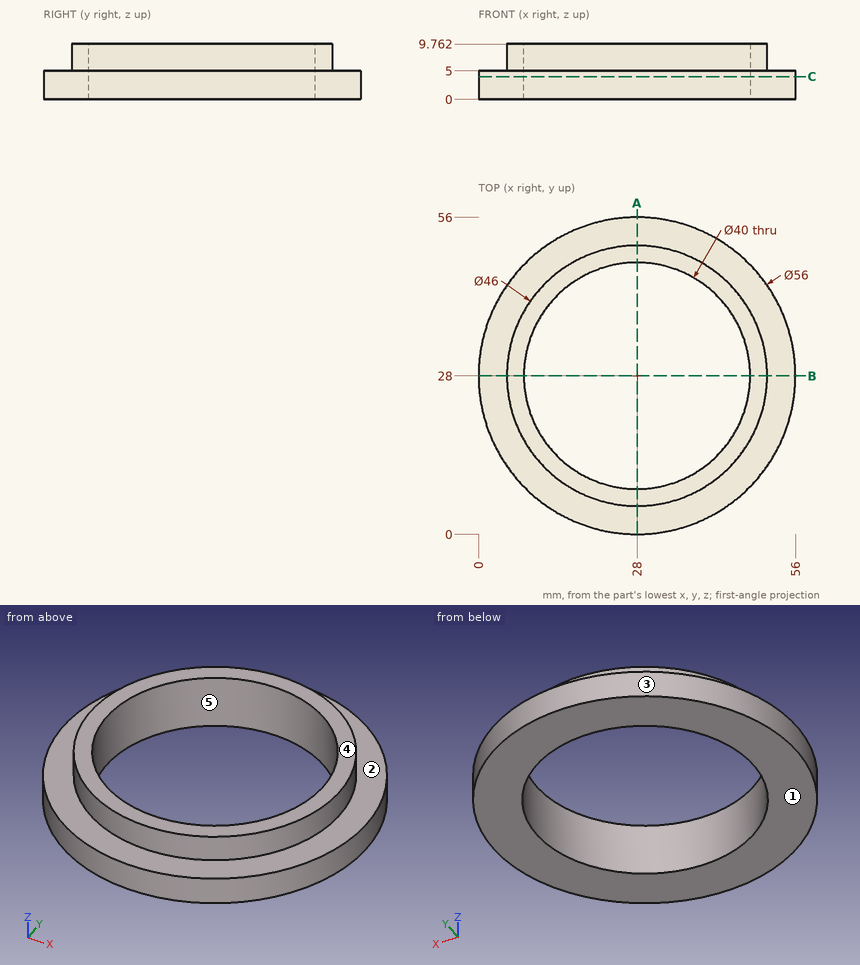
Input: dimensioned drawing with shaded views. Units: mm. Origin: part minimum x, y, z. A direction names the side the tool comes from. Round coordinates to 2 decimals unless told otherwise and drop trailing zeros. Loops run counter-clockwise (first coordinate to the right, second up) from the corner with the lowest first, then second, coordinate; pieces in that order, holes last.
1) Pull-direction query (X, two-part tool) for the marked faces 3, 4 and 5; classes: released by +X, released by -X, zero draft, split by the parting line, or undercut.
Ans:
face 3: split by the parting line
face 4: zero draft
face 5: undercut
2) Pin query (flat end, axial travel): pin 1 (1.5 mm diameter, centred on x = 28, z = 7.5, fed in from -Y); pin 2 (2 mm diameter, centred on x = 48.5, z = 1.5, fed in from -Y) (1 decimal); pin 3 (4 mm diameter, centred on y = 19.5, z = 6, fed in from +X). Return the tip coordinate at first contact, or that it passes through.
Ans:
pin 1: stops at y = 5
pin 2: stops at y = 7.9
pin 3: stops at x = 55.17
3) Material intervals for line 1 (Y direction, x = 28, z = 2.75); line 2 (Z direction, x = 12.5, y = 8); line 3 (Y direction, x = 13.5, z = 9.5) (1 decimal), sorted ascending.
Ans:
line 1: y = 0 to 8, 48 to 56
line 2: z = 0 to 5
line 3: y = 10.1 to 14.2, 41.8 to 45.9
4) Section query C-C on z = 4. Return the cut outline in (x, y).
Ans:
outline: circle Ø56 at (28, 28); hole circle Ø40 at (28, 28)
5) Section query A-A on x = 28. Return the cut outline in (y, z), plus the area to 3 significant figures.
Ans:
outline: (0, 0) - (8, 0) - (8, 9.76) - (5, 9.76) - (5, 5) - (0, 5) - close; (48, 0) - (56, 0) - (56, 5) - (51, 5) - (51, 9.76) - (48, 9.76) - close
area: 109 mm2
6) Set-up query: the marked faces 1 and 2. Return all of +Z, -Z, +X, -X, +Y, -Y with unobstructed straight access to the full face (end or side cutting, diameter ignored); none if empty.
Ans:
face 1: -Z, +X, -X, +Y, -Y
face 2: +Z
